from build123d import *

# Parameters (mm, degrees)
BOSS_EXTRUDE1_DEPTH = 2.54
SKETCH2_R           = 4.191
CUT_EXTRUDE1_DEPTH  = 95.508529347


with BuildPart() as part:
    # Sketch1 → Boss-Extrude1 (new body)
    with BuildSketch(Plane(origin=(0, 0, 0), x_dir=(0, 0, -1), z_dir=(1, 0, 0))):
        Polygon((21.030595238, 39.385119048), (48.970595238, 39.385119048), (54.050595238, 44.465119048), (54.050595238, 72.405119048), (48.970595238, 77.485119048), (-17.069404762, 77.485119048), (-22.149404762, 72.405119048), (-22.149404762, -43.164880952), (15.950595238, -43.164880952), (15.950595238, 34.305119048), align=None)
    extrude(amount=BOSS_EXTRUDE1_DEPTH)

    # Sketch2 → Cut-Extrude1 (cut, through all)
    with BuildSketch(Plane(origin=(2.54, 0, 0), x_dir=(0, 0, -1), z_dir=(1, 0, 0))):
        with Locations((-13.259404762, -24.114880952)):
            Circle(SKETCH2_R)
        with Locations((7.060595238, -24.114880952)):
            Circle(SKETCH2_R)
    extrude(amount=-CUT_EXTRUDE1_DEPTH, mode=Mode.SUBTRACT)


solid = part.part
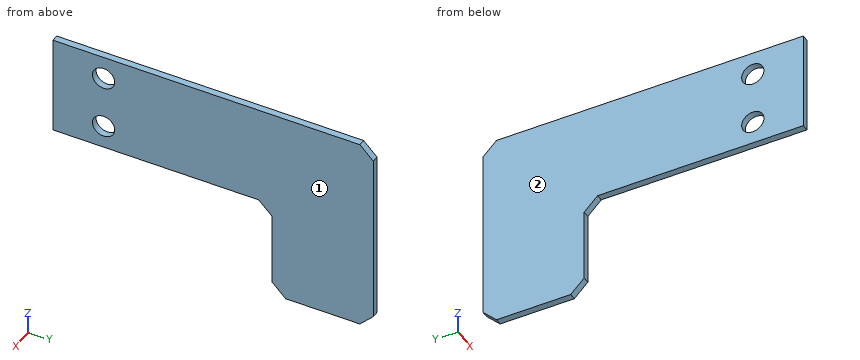
Geometry: final body of the model. Coordinates: model frame, mm. Face numbers are marked on the shaded views. Coordinates: 2 decimals unless noted, no trailing zeros. Loops run counter-clockwise (first coordinate to the right, second up) from the corner with the lowest first, then second, coordinate; pieces in that order, holes last. Notation, with made-up numbers: (52.25, -23) - (108.25, -23) arc R28 cw to (108.25, -3) - close; hole circle Ø5 at (31.25, -18.75). An arc over 180 degrees is marked (long way). One line per question, with ' | ' between items. Start each with the question number.
(1) Ray query, L1, parallel to Y at x = 1.05, z = 13.5; L2, parallel to Y at x = 1.35, z = -27.5; L3, parallel to Z at x = 1.2, y = -19. Return the intervals inside material, ascending. Write a range as from..to.
(2) Cut plane C-C on x = 1.55. Output: boundary loops of the cut face in (y, z), and give its area (3 significant figures).
(3) Draft query along X for the marked faces 1 and 2. Return one class per face: +X half, -X half, draft (parallel to the pull), parting line (faces both ways), or undercut.
(4) Cut plane B-B on z = 14. Output: boundary loops of the cut face in (x, y).
(5) Cut plane A-A on y = -22. Output: boundary loops of the cut face in (x, z).
(6) First-contact query: pin 1 (0.8 mm diameter, centred on x = 2, z = -40, fed in from -Y); pin 2 (2 mm diameter, centred on y = 43, z = -2, fed in from -X); pin 3 (0.8 mm diameter, centred on x = 1, y = -16.5, fed in from -Z). Flat tips, straight axial feed; report the tip coordinate or a pass-through.
(7) Cut plane D-D on y = 18. Output: boundary loops of the cut face in (x, z).
Here are the results:
1) L1: -43.16..-28.3, -19.93..77.49 | L2: 39.39..77.49 | L3: -15.95..22.15
2) outline: (-43.16, -15.95) - (34.31, -15.95) - (39.39, -21.03) - (39.39, -48.97) - (44.47, -54.05) - (72.41, -54.05) - (77.49, -48.97) - (77.49, 17.07) - (72.41, 22.15) - (-43.16, 22.15) - close; hole circle Ø8.38 at (-24.11, -7.06); hole circle Ø8.38 at (-24.11, 13.26) | area: 5,910 mm²
3) face 1: +X half | face 2: -X half
4) outline: (0, -43.16) - (2.54, -43.16) - (2.54, -28.24) - (0, -28.24) - close; (0, -19.99) - (2.54, -19.99) - (2.54, 77.49) - (0, 77.49) - close
5) outline: (0, -15.95) - (2.54, -15.95) - (2.54, -10.68) - (0, -10.68) - close; (0, -3.44) - (2.54, -3.44) - (2.54, 9.64) - (0, 9.64) - close; (0, 16.88) - (2.54, 16.88) - (2.54, 22.15) - (0, 22.15) - close
6) pin 1: y = 39.39 | pin 2: x = 0 | pin 3: z = -15.95
7) outline: (0, -15.95) - (2.54, -15.95) - (2.54, 22.15) - (0, 22.15) - close
